The listing builds one solid part. Answer for the finished solid, in the listing's coordinates (mm). Face numbers are marked on the shaded views. A direction names the side the tool comes from. Round coordinates to 2 decimals unless told otherwise and drop trailing zeros. Loops run counter-clockwise (first coordinate to the right, second up) from the corner with the lowest first, then second, coordinate; pieces in that order, holes last. Notation, with made-up numbers: M 35.5,37.5 L 55.5,37.5 A29 cw 55.5,63.5 Z; hole C 21.5,-28.5 d11. An arc over 180 degrees is marked long. Put each result on its own line as item: value. Start each with the question number.
(1) Section A-A, the plane x = 76.2 is taken. Determine the outline of the cut face in (y, z), then the cut area to 3 significant figures.
(2) Section D-D, the plane z = 19.5 is taken. Determine the outline of the cut face in (x, y), then the cut area to 3 significant figures.
(3) Section C-C, the plane z = -41 is taken. Determine the outline of the cut face in (x, y).
(4) Straight lines are drawn through the part: line 1 (X direction, y = -12, z = -35); line 2 (Y direction, x = 25, z = -40); line 3 (Y direction, x = 76.2, z = -21). For each, find the intervals that lie inside material, in ascending order.
(5) Flat-ended cylindrical pins translate along their axes: P1, Ø4, axis at x = 119, y = -45, coming from the +Z side; P2, Ø6, axis at y = -39.5, z = -43, coming from the -X side; P3, Ø11, axis at x = 76.2, y = -12.7, coming from the +Z side (3 decimals). Find the tip coordinate at first contact, or state that the pin passes through.
(6) Which of the six approach directions +Z, -Z, +X, -X, +Y, -Y give full straight-line access (tool end or side, diameter ignored) to the marked faces 1, 2 and 3?
(7) Section B-B, the plane y = -12.7 is taken. Determine the outline of the cut face in (x, z), then the cut area to 3 significant figures.
```python
from build123d import *

# Parameters (mm, degrees)
F1_DEPTH    = 25.4
F2_R        = 5.8227150046
F2_R_2      = 6.8159523424
F3_DEPTH    = 152.4
F4_W        = 99.5925068855
F4_H        = 61.3070130348
F5_DEPTH    = 25.4
F6_T1_DEPTH = 61.3070130348
F7_R        = 5.08
F8_R        = 5.08
F9_R        = 5.08
F10_R       = 5.08
F11_R       = 5.08
F12_R       = 5.08
F13_R       = 5.08


# Not quite as in the source:
# - a fillet or chamfer that OpenCascade refuses, or shapes differently, is made with other operations: its cross-section is extruded or revolved along the edge and cut away or added


with BuildPart() as f1:
    # F0 (on Front) → F1 (new body)
    with BuildSketch(Plane.XZ):
        Polygon((118.0045455694, 0), (0, 0), (0, -61.3070130348), (217.5970524549, -61.3070130348), (217.5970524549, 84.4091549516), (118.0045455694, 84.4091549516), align=None)
    extrude(amount=F1_DEPTH)

    # F2 (on face) → F3 (cut)
    with BuildSketch(Plane.XY):
        with Locations((25.4, -12.7)):
            Circle(F2_R)
        with Locations((76.2, -12.7)):
            Circle(F2_R_2)
    extrude(amount=-F3_DEPTH, mode=Mode.SUBTRACT)

    # F4 (on face) → F5 (join)
    with BuildSketch(Plane.XZ.offset(25.4)):
        with Locations((167.8007990122, -30.6535065174)):
            Rectangle(F4_W, F4_H)
    extrude(amount=F5_DEPTH)

    # F6: fillet of radius 5.08 on 1 edges, made by hand

    # F6_s2 → F6_t1 (join)
    with BuildSketch(Plane.XY.offset(-61.3070130348)):
        with BuildLine():
            ThreePointArc((118.0045455694, -30.48), (116.5166480178, -26.8878975516), (112.9245455694, -25.4))
            Line((112.9245455694, -25.4), (118.0045455694, -25.4))
            Line((118.0045455694, -25.4), (118.0045455694, -30.48))
        make_face()
    extrude(amount=F6_T1_DEPTH)

    # F7
    f7_edges = [f1.edges().sort_by_distance(p)[0] for p in [
        (118.004546, -25.4, 42.204577),
    ]]
    fillet(f7_edges, radius=F7_R)

    # F8
    f8_edges = [f1.edges().sort_by_distance(p)[0] for p in [
        (217.597052, -25.4, 42.204577),
    ]]
    fillet(f8_edges, radius=F8_R)

    # F9
    f9_edges = [f1.edges().sort_by_distance(p)[0] for p in [
        (217.597052, -38.1, 0),
        (217.597052, -50.8, -30.653507),
    ]]
    fillet(f9_edges, radius=F9_R)

    # F10
    f10_edges = [f1.edges().sort_by_distance(p)[0] for p in [
        (217.597052, -22.86, -61.307013),
    ]]
    fillet(f10_edges, radius=F10_R)

    # F11
    f11_edges = [f1.edges().sort_by_distance(p)[0] for p in [
        (217.597052, 0, 14.091071),
    ]]
    fillet(f11_edges, radius=F11_R)

    # F12
    f12_edges = [f1.edges().sort_by_distance(p)[0] for p in [
        (118.004546, 0, 42.204577),
    ]]
    fillet(f12_edges, radius=F12_R)

    # F13
    f13_edges = [f1.edges().sort_by_distance(p)[0] for p in [
        (0, 0, -28.113507),
        (0, -1.487898, -59.819115),
        (0, -15.24, -61.307013),
    ]]
    fillet(f13_edges, radius=F13_R)


solid = f1.part
```
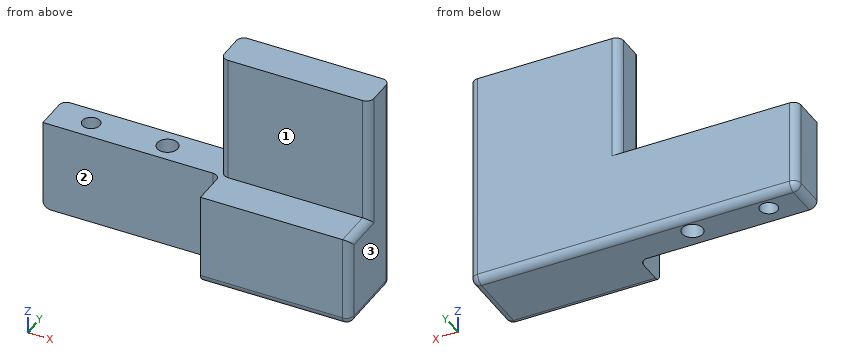
Recorded:
1. outline: M -25.4,-61.31 L -19.52,-61.31 L -19.52,0 L -25.4,0 Z; M -5.88,-61.31 L -5.08,-61.31 A5.08 ccw 0,-56.23 L 0,0 L -5.88,0 Z
1. area: 716 mm²
2. outline: M 118,-20.32 A5.08 ccw 123.08,-25.4 L 212.52,-25.4 A5.08 ccw 217.6,-20.32 L 217.6,-5.08 A5.08 ccw 212.52,0 L 123.08,0 A5.08 ccw 118,-5.08 Z
2. area: 2,510 mm²
3. outline: M 0,-25.4 L 112.92,-25.4 A5.08 cw 118,-30.48 L 118,-50.8 L 212.52,-50.8 A5.08 ccw 217.6,-45.72 L 217.6,-5.08 A5.08 ccw 212.52,0 L 5.08,0 A5.08 ccw 0,-5.08 Z; hole C 25.4,-12.7 d11.65; hole C 76.2,-12.7 d13.63
4. line 1: x = 0 to 19.62, 31.18 to 69.42, 82.98 to 217.6
4. line 2: y = -25.4 to -18.51, -6.89 to 0
4. line 3: y = -25.4 to -19.52, -5.88 to 0
5. P1: stops at z = 0
5. P2: stops at x = 118
5. P3: passes through
6. face 1: +Z, +X, -X, -Y
6. face 2: +Z, -Z, -X, -Y
6. face 3: +Z, -Z, +X, +Y, -Y
7. outline: M 0,-56.23 A5.08 ccw 5.08,-61.31 L 19.58,-61.31 L 19.58,0 L 0,0 Z; M 31.22,-61.31 L 69.38,-61.31 L 69.38,0 L 31.22,0 Z; M 83.02,-61.31 L 212.52,-61.31 A5.08 ccw 217.6,-56.23 L 217.6,84.41 L 118,84.41 L 118,0 L 83.02,0 Z
7. area: 20,200 mm²
